Input: part model. Units: mm. Frame: model coordinates. A direction names the side the tool comes from. Round coordinates to 2 decimals unless told otherwise and drop trailing zeros. Order: outer loops, then holes, each group sorted by start corner. A loop starts at its lowest first (then second) coordinate and runs counter-clockwise, first axis right, second up. Notation, with made-up numbers: (74, 16) -> (121, 16) arc R18 ccw to (121, 31) -> close; hole circle Ø10 at (1, 76.5). An arc over 180 degrees is marked (long way). Answer as CSV lines item,"result". Start each with the question number.
1) First-contact query: P1, Ø0.8, axis at y = -14, z = -2.5, coming from the +X side; P2, Ø2, axis at y = -13.5, z = 4, coming from the -X side; P3, Ø10, axis at x = -5.5, z = 2.5, coming from the +Y side; P4, Ø10, axis at x = 7, y = 0.5, coming from the +Z side. Flat tips, straight axial feed; report the tip coordinate or a pass-through.
2) Mould query, pull axis X, two halves, no side actions, for faces 1 (the face through (-34.29, 3, 7)), 2 (the face through (-10.16, -5.1, 6.6)), 3 (the face through (0, -15.24, 11)). Classes: +X half, -X half, draft (parallel to the pull), parting line (faces both ways), or undercut.
3) Access query for faces 4 (the face through (0, -14, -9.525)), 5 (the face through (-29.21, -13, 6)), 6 (the face through (29.21, -13, 6)), 7 (the face through (14, 0, 0)), 8 (the face through (0, -12.7, 11)). Directions: +Z, -Z, +X, -X, +Y, -Y. A direction counts if a zero-diameter tool reaches every point of the face in a straight line with its end or side. Return the directions, or none.
4) Section query B-B, the plane x = 15. Output: boundary loops of the cut face in (y, z), and give its area (3 significant figures).
5) Line query: L1, parallel to X at y = -6, z = 3.5; L2, parallel to X at y = -11, z = 12; L3, parallel to Y at x = 7, z = -6. Output: solid intervals per line, ascending.
6) Section query A-A, the plane x = -5.5. Output: boundary loops of the cut face in (y, z) (3 decimals), and give its area (3 significant figures).
```python
from build123d import *

# Parameters (mm, degrees)
SKETCH1_W               = 50.8
SKETCH1_H               = 30.48
BOSS_EXTRUDE1_DEPTH     = 34.29
SKETCH2_R               = 18.034
CUT_EXTRUDE1_DEPTH      = 46.312489448
SKETCH3_W               = 20.32
SKETCH3_H               = 27.94
CUT_EXTRUDE2_DEPTH      = 64.156169137
SKETCH4_W               = 12.7
SKETCH4_H               = 19.05
CUT_EXTRUDE3_DEPTH      = 46.312489448
SKETCH7_W               = 68.58
SKETCH7_H               = 12.7
CUT_EXTRUDE5_DEPTH      = 53.440389968
CUT_EXTRUDE6_DEPTH      = 46.312489448
CUT_EXTRUDE6_DEPTH_BACK = 46.312489448
SKETCH9_W               = 5.08
SKETCH9_H               = 5.08


with BuildPart() as part:
    # Sketch1 → Boss-Extrude1 (new, symmetric)
    with BuildSketch(Plane(origin=(0, 0, 0), x_dir=(0, 0, -1), z_dir=(1, 0, 0))):
        Rectangle(SKETCH1_W, SKETCH1_H)
    extrude(amount=BOSS_EXTRUDE1_DEPTH, both=True)

    # Sketch2 → Cut-Extrude1 (cut, through all)
    with BuildSketch(Plane(origin=(0, 0, 0), x_dir=(1, 0, 0), z_dir=(0, 0.819152044288991, 0.5735764363510473))):
        with Locations(Location((0, 0, 0), (0, 0, 221.991688173))):
            Circle(SKETCH2_R)
    extrude(amount=CUT_EXTRUDE1_DEPTH, mode=Mode.SUBTRACT)

    # Sketch3 → Cut-Extrude2 (cut, through all)
    with BuildSketch(Plane.XY.offset(25.4)):
        with Locations((0, 1.27)):
            Rectangle(SKETCH3_W, SKETCH3_H)
    extrude(amount=-CUT_EXTRUDE2_DEPTH, mode=Mode.SUBTRACT)

    # Sketch4 → Cut-Extrude3 (cut, through all)
    with BuildSketch(Plane(origin=(0, 0, 0), x_dir=(1, 0, 0), z_dir=(0, 1, 0))):
        Rectangle(SKETCH4_W, SKETCH4_H)
    extrude(amount=-CUT_EXTRUDE3_DEPTH, mode=Mode.SUBTRACT)

    # Sketch7 → Cut-Extrude5 (cut, through all)
    with BuildSketch(Plane(origin=(0, 15.24, 0), x_dir=(1, 0, 0), z_dir=(0, 1, 0))):
        with Locations((0, 19.05)):
            Rectangle(SKETCH7_W, SKETCH7_H)
    extrude(amount=-CUT_EXTRUDE5_DEPTH, mode=Mode.SUBTRACT)

    # Sketch9 → Cut-Extrude6 (cut, two sides: drawn at the far end of the back side and taken through both)
    with BuildSketch(Plane.XY.offset(-CUT_EXTRUDE6_DEPTH_BACK)):
        with Locations((-31.75, -12.7)):
            Rectangle(SKETCH9_W, SKETCH9_H)
        with Locations((31.75, -12.7)):
            Rectangle(SKETCH9_W, SKETCH9_H)
    extrude(amount=CUT_EXTRUDE6_DEPTH + CUT_EXTRUDE6_DEPTH_BACK, mode=Mode.SUBTRACT)


solid = part.part
```
Findings:
1,P1,"stops at x = 29.21"
1,P2,"stops at x = -29.21"
1,P3,"stops at y = -0.48"
1,P4,"stops at z = 25.4"
2,face 1,"-X half"
2,face 2,"undercut"
2,face 3,"draft"
3,face 4,"+Y, -Y"
3,face 5,"+Z, -Z, -X, -Y"
3,face 6,"+Z, -Z, +X, -Y"
3,face 7,"none"
3,face 8,"+Z, -Z, +Y"
4,outline,"(-15.24, -12.7) -> (15.24, -12.7) -> (15.24, -1.55) -> (5.74, -8.2) -> (-5.74, 8.2) -> (15.24, 22.89) -> (15.24, 25.4) -> (-15.24, 25.4) -> close"
4,area,"789 mm^2"
5,L1,"x = -34.29 to -10.16, 10.16 to 34.29"
5,L2,"x = -29.21 to -10.16, 10.16 to 29.21"
5,L3,"y = -15.24 to -12.7"
6,outline,"(-15.24, -12.7) -> (-12.7, -12.7) -> (-12.7, -9.525) -> (-15.24, -9.525) -> close; (-15.24, 9.525) -> (-12.7, 9.525) -> (-12.7, 25.4) -> (-15.24, 25.4) -> close"
6,area,"48.4 mm^2"
